Read the model definition and answer for the solid it produces. Units are mm, in the model's axes. Face numbers are marked on the shaded views. A direction names the side the tool comes from. Coordinates: 2 decimals unless noted, no trailing zeros. Order: outer loops, then holes, each group sorted by start corner. A loop starts at its lowest first (then second) coordinate and runs counter-clockwise, first axis right, second up.
Autodesk Inventor part; units mm, degrees
ref_plane "YZ Plane" through (0, 0, 0) normal (1, 0, 0) x (0, 1, 0)
ref_plane "XZ Plane" through (0, 0, 0) normal (0, 1, 0) x (-1, 0, 0)
ref_plane "XY Plane" through (0, 0, 0) normal (0, 0, 1) x (1, 0, 0)
sketch "Sketch1" plane through (0, 0, 0) normal (0, 0, 1) x (1, 0, 0)
  line L0 (0, 0) -> (3.175, 0)
  line L1 (3.175, 0) -> (3.175, 25.4)
  line L2 (3.175, 25.4) -> (0, 25.4)
  line L3 (0, 25.4) -> (0, 0)
  line L4 (0, 0) -> (25.4, 0)
  line L5 (25.4, 0) -> (25.4, 3.175)
  line L6 (25.4, 3.175) -> (0, 3.175)
  line L7 (0, 3.175) -> (0, 0)
  dimension "d0" = 3.175
  dimension "d1" = 25.4
  dimension "d2" = 25.4
  dimension "d3" = 3.175
extrude "Extrusion1" add sketch "Sketch1" along normal blind 25.4
sketch "Sketch2" plane through (3.175, 3.175, 0) normal (0, 1, 0) x (1, 0, 0)
  line L0 (22.225, 0) -> (0, 0) construction
  line L1 (11.1125, 0) -> (11.1125, -12.7) construction
  line L2 (11.1125, 0) -> (23.8125, 0) construction
  circle A0 centre (11.1125, -12.7) radius 1.9812
  point P0 (-3.175, 0)
  dimension "d6" = 12.7
  dimension "d7" = 90
  dimension "d8" = 3.9624
extrude "Extrusion2" cut sketch "Sketch2" against normal blind 25.4
sketch "Sketch3" plane through (3.175, 3.175, 0) normal (1, 0, 0) x (0, 0, -1)
  line L0 (0, 22.225) -> (-25.4, 22.225) construction
  circle A0 centre (-12.7, 9.525) radius 2.5797
  line L1 (-12.7, 9.525) -> (-12.7, 22.225)
  point P0 (0, -3.175)
  dimension "d11" = 5.1594
  dimension "d14" = 12.7
extrude "Extrusion3" cut sketch "Sketch3" against normal blind 25.4
properties part number "L-Bracket Bumper"
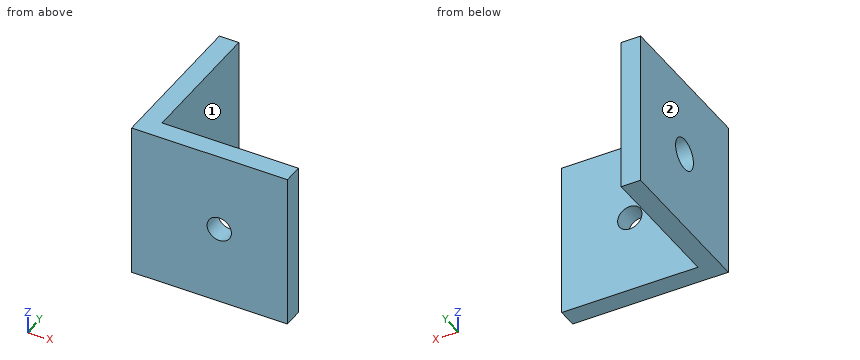
1) A cutting plane is placed at A-A, the plane z = 12.7. Determine the outline of the cut face in (x, y) (3 decimals), and give its area (3 significant figures).
A:
outline: (0, 0) - (12.306, 0) - (12.306, 3.175) - (3.175, 3.175) - (3.175, 10.12) - (0, 10.12) - close; (0, 15.28) - (3.175, 15.28) - (3.175, 25.4) - (0, 25.4) - close; (16.269, 0) - (25.4, 0) - (25.4, 3.175) - (16.269, 3.175) - close
area: 122 mm2
2) A cutting plane is placed at B-B, the plane y = 12.7. Determine the outline of the cut face in (x, z) (3 decimals), and give its area (3 significant figures).
A:
outline: (0, 0) - (3.175, 0) - (3.175, 10.12) - (0, 10.12) - close; (0, 15.28) - (3.175, 15.28) - (3.175, 25.4) - (0, 25.4) - close
area: 64.3 mm2
3) A cutting plane is placed at C-C, the plane z = 19.75. Determine the outline of the cut face in (x, y) (3 decimals), and give its area (3 significant figures).
A:
outline: (0, 0) - (25.4, 0) - (25.4, 3.175) - (3.175, 3.175) - (3.175, 25.4) - (0, 25.4) - close
area: 151 mm2
4) Which of the six approach directions +Z, -Z, +X, -X, +Y, -Y give full straight-line access (tool end or side, diameter ignored) to the marked faces 1 and 2?
A:
face 1: +Z, -Z, +X, +Y
face 2: +Z, -Z, -X, +Y, -Y
5) Straight lines are drawn through the part: line 1 (X direction, y = 3, z = 12.75); line 2 (Y direction, x = 1.6, z = 12.7); line 3 (X direction, y = 5.25, z = 1) (3 decimals). For each, find the intervals that lie inside material, in ascending order.
A:
line 1: x = 0 to 12.31, 16.27 to 25.4
line 2: y = 0 to 10.12, 15.28 to 25.4
line 3: x = 0 to 3.175
6) Flat-ended cylindrical pins translate along their axes: pin 1 Ø8 at (y, z) = (14, 5) entering from +X (3 decimals); pin 2 Ø5 at (x, z) = (17.5, 18.5) entering from +Y (3 decimals); pin 3 Ø3 at (x, z) = (14.29, 12.7) entering from +Y. Find the tip coordinate at first contact, or state that the pin passes through.
A:
pin 1: stops at x = 3.175
pin 2: stops at y = 3.175
pin 3: passes through
7) A cutting plane is placed at D-D, the plane y = 20.75. Determine the outline of the cut face in (x, z) (3 decimals), and give its area (3 significant figures).
A:
outline: (0, 0) - (3.175, 0) - (3.175, 25.4) - (0, 25.4) - close
area: 80.6 mm2
